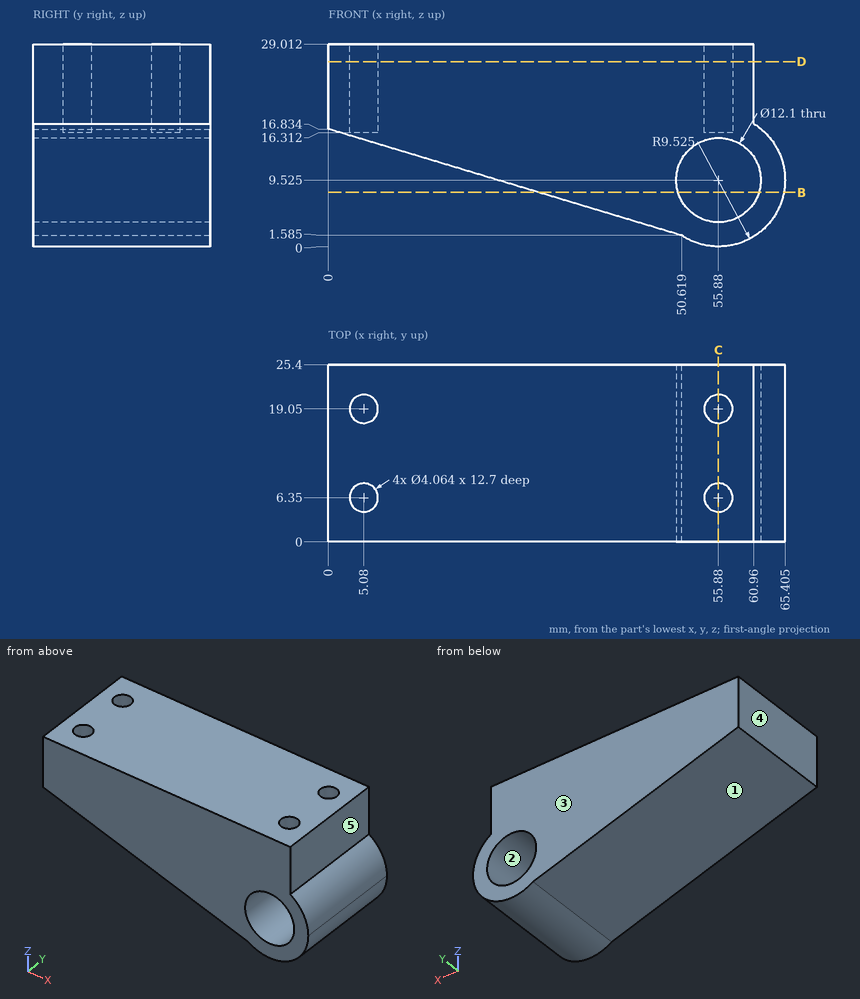
Design review of the part shown in the three views and the two pictorial views. Dimensions are in mm from the part's minimum x, y and z. A direction names the side the tool comes from. Round coordinates to 2 decimals unless told otherwise and drop trailing zeros. Write each loop counter-clockwise with the first axis right and the second up, starting at its lowest first coordinate (ties: lowest second). Pieces come first, ordered by that corner, then holes. Notation, with made-up numbers: (64.5, 9) -> (108.5, 9) arc R15 cw to (108.5, 20) -> close; hole circle Ø2 at (32.25, 83). An arc over 180 degrees is marked (long way). Use one line per item in the form item = value.
1) Take a section at B-B, the plane z = 7.75. Write out the cut boundary in (x, y), and give its area (3 significant figures).
Found:
outline = (30.15, 0) -> (50.1, 0) -> (50.1, 25.4) -> (30.15, 25.4) -> close; (61.66, 0) -> (65.24, 0) -> (65.24, 25.4) -> (61.66, 25.4) -> close
area = 597 mm2
2) Mouldability with a two-part tool opening along X and no side actions: class the marked faces 1, 2 and 3 as +X half, -X half, draft (parallel to the pull), parting line (faces both ways), or undercut.
Found:
face_1 = -X half
face_2 = undercut
face_3 = draft
3) Take a section at D-D, the plane z = 26.5. Write out the cut boundary in (x, y).
Found:
outline = (0, 0) -> (60.96, 0) -> (60.96, 25.4) -> (0, 25.4) -> close; hole circle Ø4.06 at (5.08, 6.35); hole circle Ø4.06 at (5.08, 19.05); hole circle Ø4.06 at (55.88, 6.35); hole circle Ø4.06 at (55.88, 19.05)
4) Take a section at C-C, the plane x = 55.88. Write out the cut boundary in (y, z) (1 decimal).
Found:
outline = (0, 0) -> (25.4, 0) -> (25.4, 3.5) -> (0, 3.5) -> close; (0, 15.6) -> (25.4, 15.6) -> (25.4, 29) -> (21.1, 29) -> (21.1, 16.3) -> (17, 16.3) -> (17, 29) -> (8.4, 29) -> (8.4, 16.3) -> (4.3, 16.3) -> (4.3, 29) -> (0, 29) -> close
5) To check wall thickness, follow L1, parallel to Y at x = 5.08, z = 23.25; L2, parallel to X at y = 14.5, z = 26.5; L3, parallel to Z at x = 59, y = 23.5 (1 decimal). State the ranges of each line that lie inside material, in increasing order. Write a range as from..to.
Found:
L1 = 0..4.32, 8.38..17.02, 21.08..25.4
L2 = 0..60.96
L3 = 0.5..4.3, 14.7..29
6) Tool access review of the marked faces 4 and 5: name each direction out of +Z, -Z, +X, -X, +Y, -Y from which nothing blocks a thin tool from reaching the whole face with its end or side.
Found:
face_4 = +Z, -Z, -X, +Y, -Y
face_5 = +Z, +X, +Y, -Y
7) Clearance check with flat-ended pins moving along their axes: pin 1 (1.5 mm diameter, centred on y = 7.5, z = 25.5, fed in from +X); pin 2 (8 mm diameter, centred on y = 14.5, z = 21, fed in from +X); pin 3 (4.5 mm diameter, centred on x = 5.08, y = 19.05, fed in from -Z) (1 decimal). State where each tip first meets the part, or that it passes through.
Found:
pin_1 = 60.96
pin_2 = 61.78
pin_3 = 14.6
